from build123d import *

# Parameters (mm, degrees)
SKETCH2_W               = 65
SKETCH2_H               = 37.5
SKETCH2_R               = 1.6
SKETCH2_R_2             = 0.201294772
BOSS_EXTRUDE1_DEPTH     = 2
SKETCH2_3_R             = 0.505
BOSS_EXTRUDE2_DEPTH     = 0.1
LPATTERN1_COUNT         = 8
LPATTERN1_PITCH         = 2.54
MIRROR1_COPY_1_SKETCH_R = 0.505
MIRROR1_COPY_1_DEPTH    = 0.1
MIRROR1_COPY_2_SKETCH_R = 0.505
MIRROR1_COPY_2_DEPTH    = 0.1
MIRROR1_COPY_3_SKETCH_R = 0.505
MIRROR1_COPY_3_DEPTH    = 0.1
MIRROR1_COPY_4_SKETCH_R = 0.505
MIRROR1_COPY_4_DEPTH    = 0.1
MIRROR1_COPY_5_SKETCH_R = 0.505
MIRROR1_COPY_5_DEPTH    = 0.1
MIRROR1_COPY_6_SKETCH_R = 0.505
MIRROR1_COPY_6_DEPTH    = 0.1
MIRROR1_COPY_7_SKETCH_R = 0.505
MIRROR1_COPY_7_DEPTH    = 0.1
MIRROR2_COPY_1_SKETCH_R = 0.505
MIRROR2_COPY_1_DEPTH    = 0.1
MIRROR2_COPY_2_SKETCH_R = 0.505
MIRROR2_COPY_2_DEPTH    = 0.1
MIRROR2_COPY_3_SKETCH_R = 0.505
MIRROR2_COPY_3_DEPTH    = 0.1
MIRROR2_COPY_4_SKETCH_R = 0.505
MIRROR2_COPY_4_DEPTH    = 0.1
MIRROR2_COPY_5_SKETCH_R = 0.505
MIRROR2_COPY_5_DEPTH    = 0.1
MIRROR2_COPY_6_SKETCH_R = 0.505
MIRROR2_COPY_6_DEPTH    = 0.1
MIRROR2_COPY_7_SKETCH_R = 0.505
MIRROR2_COPY_7_DEPTH    = 0.1


with BuildPart() as part:
    # Sketch2 → Boss-Extrude1 (new body)
    with BuildSketch(Plane.XY):
        with Locations((0.820647671, -17.581573661)):
            Rectangle(SKETCH2_W, SKETCH2_H)
        with Locations((30.570647671, -1.431573661)):
            Circle(SKETCH2_R, mode=Mode.SUBTRACT)
        with Locations((30.570647671, -33.581573661)):
            Circle(SKETCH2_R, mode=Mode.SUBTRACT)
        with Locations((-28.679352329, -1.431573661)):
            Circle(SKETCH2_R, mode=Mode.SUBTRACT)
        with Locations((-28.979352329, -33.431573661)):
            Circle(SKETCH2_R, mode=Mode.SUBTRACT)
        with Locations((29.137165251, -7.831573661)):
            Circle(SKETCH2_R_2, mode=Mode.SUBTRACT)
    extrude(amount=-BOSS_EXTRUDE1_DEPTH)

    # Sketch2<3> → Boss-Extrude2 (add)
    with BuildSketch(Plane.XY):
        with Locations((31.770647671, -7.831573661)):
            Circle(SKETCH2_3_R)
    boss_extrude2 = extrude(amount=BOSS_EXTRUDE2_DEPTH)

    # LPattern1: Boss-Extrude2 ×8
    with Locations(*[(0, -i * LPATTERN1_PITCH, 0) for i in range(1, LPATTERN1_COUNT)]):
        add(boss_extrude2)

    # Mirror1: Boss-Extrude2 across plane
    add(boss_extrude2.mirror(Plane(origin=(30.453906461, 0, 0), x_dir=(0, 0, 1), z_dir=(1, 0, 0))))

    # Mirror1 copy 1 sketch → Mirror1 copy 1 (add)
    with BuildSketch(Plane(origin=(60.907812922, -2.54, 0), x_dir=(-1, 0, 0), z_dir=(0, 0, 1))):
        with Locations((31.770647671, 7.831573661)):
            Circle(MIRROR1_COPY_1_SKETCH_R)
    extrude(amount=MIRROR1_COPY_1_DEPTH)

    # Mirror1 copy 2 sketch → Mirror1 copy 2 (add)
    with BuildSketch(Plane(origin=(60.907812922, -5.08, 0), x_dir=(-1, 0, 0), z_dir=(0, 0, 1))):
        with Locations((31.770647671, 7.831573661)):
            Circle(MIRROR1_COPY_2_SKETCH_R)
    extrude(amount=MIRROR1_COPY_2_DEPTH)

    # Mirror1 copy 3 sketch → Mirror1 copy 3 (add)
    with BuildSketch(Plane(origin=(60.907812922, -7.62, 0), x_dir=(-1, 0, 0), z_dir=(0, 0, 1))):
        with Locations((31.770647671, 7.831573661)):
            Circle(MIRROR1_COPY_3_SKETCH_R)
    extrude(amount=MIRROR1_COPY_3_DEPTH)

    # Mirror1 copy 4 sketch → Mirror1 copy 4 (add)
    with BuildSketch(Plane(origin=(60.907812922, -10.16, 0), x_dir=(-1, 0, 0), z_dir=(0, 0, 1))):
        with Locations((31.770647671, 7.831573661)):
            Circle(MIRROR1_COPY_4_SKETCH_R)
    extrude(amount=MIRROR1_COPY_4_DEPTH)

    # Mirror1 copy 5 sketch → Mirror1 copy 5 (add)
    with BuildSketch(Plane(origin=(60.907812922, -12.7, 0), x_dir=(-1, 0, 0), z_dir=(0, 0, 1))):
        with Locations((31.770647671, 7.831573661)):
            Circle(MIRROR1_COPY_5_SKETCH_R)
    extrude(amount=MIRROR1_COPY_5_DEPTH)

    # Mirror1 copy 6 sketch → Mirror1 copy 6 (add)
    with BuildSketch(Plane(origin=(60.907812922, -15.24, 0), x_dir=(-1, 0, 0), z_dir=(0, 0, 1))):
        with Locations((31.770647671, 7.831573661)):
            Circle(MIRROR1_COPY_6_SKETCH_R)
    extrude(amount=MIRROR1_COPY_6_DEPTH)

    # Mirror1 copy 7 sketch → Mirror1 copy 7 (add)
    with BuildSketch(Plane(origin=(60.907812922, -17.78, 0), x_dir=(-1, 0, 0), z_dir=(0, 0, 1))):
        with Locations((31.770647671, 7.831573661)):
            Circle(MIRROR1_COPY_7_SKETCH_R)
    extrude(amount=MIRROR1_COPY_7_DEPTH)

    # Mirror2: Boss-Extrude2 across plane
    add(boss_extrude2.mirror(Plane(origin=(0.82462639, 0, 0), x_dir=(0, 0, 1), z_dir=(1, 0, 0))))

    # Mirror2 copy 1 sketch → Mirror2 copy 1 (add)
    with BuildSketch(Plane(origin=(1.64925278, -2.54, 0), x_dir=(-1, 0, 0), z_dir=(0, 0, 1))):
        with Locations((31.770647671, 7.831573661)):
            Circle(MIRROR2_COPY_1_SKETCH_R)
    extrude(amount=MIRROR2_COPY_1_DEPTH)

    # Mirror2 copy 2 sketch → Mirror2 copy 2 (add)
    with BuildSketch(Plane(origin=(1.64925278, -5.08, 0), x_dir=(-1, 0, 0), z_dir=(0, 0, 1))):
        with Locations((31.770647671, 7.831573661)):
            Circle(MIRROR2_COPY_2_SKETCH_R)
    extrude(amount=MIRROR2_COPY_2_DEPTH)

    # Mirror2 copy 3 sketch → Mirror2 copy 3 (add)
    with BuildSketch(Plane(origin=(1.64925278, -7.62, 0), x_dir=(-1, 0, 0), z_dir=(0, 0, 1))):
        with Locations((31.770647671, 7.831573661)):
            Circle(MIRROR2_COPY_3_SKETCH_R)
    extrude(amount=MIRROR2_COPY_3_DEPTH)

    # Mirror2 copy 4 sketch → Mirror2 copy 4 (add)
    with BuildSketch(Plane(origin=(1.64925278, -10.16, 0), x_dir=(-1, 0, 0), z_dir=(0, 0, 1))):
        with Locations((31.770647671, 7.831573661)):
            Circle(MIRROR2_COPY_4_SKETCH_R)
    extrude(amount=MIRROR2_COPY_4_DEPTH)

    # Mirror2 copy 5 sketch → Mirror2 copy 5 (add)
    with BuildSketch(Plane(origin=(1.64925278, -12.7, 0), x_dir=(-1, 0, 0), z_dir=(0, 0, 1))):
        with Locations((31.770647671, 7.831573661)):
            Circle(MIRROR2_COPY_5_SKETCH_R)
    extrude(amount=MIRROR2_COPY_5_DEPTH)

    # Mirror2 copy 6 sketch → Mirror2 copy 6 (add)
    with BuildSketch(Plane(origin=(1.64925278, -15.24, 0), x_dir=(-1, 0, 0), z_dir=(0, 0, 1))):
        with Locations((31.770647671, 7.831573661)):
            Circle(MIRROR2_COPY_6_SKETCH_R)
    extrude(amount=MIRROR2_COPY_6_DEPTH)

    # Mirror2 copy 7 sketch → Mirror2 copy 7 (add)
    with BuildSketch(Plane(origin=(1.64925278, -17.78, 0), x_dir=(-1, 0, 0), z_dir=(0, 0, 1))):
        with Locations((31.770647671, 7.831573661)):
            Circle(MIRROR2_COPY_7_SKETCH_R)
    extrude(amount=MIRROR2_COPY_7_DEPTH)


solid = part.part
Read the model definition and answer for the solid it produces. Units are mm, in the model's axes. Round coordinates to 2 decimals unless told otherwise and drop trailing zeros. Write each loop counter-clockwise with the first axis right and the second up, starting at its lowest first coordinate (ties: lowest second). Pieces come first, ordered by that corner, then holes.
1. Given pin 1 Ø5 at (x, y) = (-28.98, -33.43) entering from +Z; pin 2 Ø2.5 at (x, y) = (30.57, -1.43) entering from -Z, each flat-ended and moving along its own axis, determine where each tip first touches the part or whether it passes through.
2. The part is cut by section B-B, the plane x = -23.5. Determine the outline of the cut face in (y, z).
3. Straight lines are drawn through the part: L1, parallel to Y at x = -29, z = -1.65; L2, parallel to Z at x = -9.5, y = -20.5. For each, find the intervals that lie inside material, in ascending order.
4. The part is cut by section A-A, the plane y = -29.5. Determine the outline of the cut face in (x, z), then the cut area to 3 significant figures.
5. Determine the mould class of faces 1 (the face through (0, 1.168, -1)), 2 (the face through (-27.153, -0.951, -0.986)), 3 (the face through (-29.188, -31.845, -0.986)), 4 (the face through (-31.679, -18, -1)) for opening direction Y: pulls with the +Y half, pulls with the -Y half, needs draft (parallel to the pull), parting line crosses it, or undercut.
Values:
1. pin 1: stops at z = 0
1. pin 2: passes through
2. outline: (-36.33, -2) - (1.17, -2) - (1.17, 0) - (-36.33, 0) - close
3. L1: y = -36.33 to -35.03, -31.83 to -3, 0.14 to 1.17
3. L2: z = -2 to 0
4. outline: (-31.68, -2) - (33.32, -2) - (33.32, 0) - (-31.68, 0) - close
4. area: 130 mm2
5. face 1: pulls with the +Y half
5. face 2: undercut
5. face 3: undercut
5. face 4: needs draft
